```python
from build123d import *

# Parameters (mm, degrees)
F0_W     = 60
F0_H     = 15
F0_H_2   = 45
F1_DEPTH = 10
F2_DEPTH = 25
F3_DEPTH = 15
F0_W_2   = 15
F4_DEPTH = 15
F5_W     = 15
F5_H     = 15
F6_DEPTH = 20
F8_DEPTH = 40


with BuildPart() as f1:
    # F0 (on Top) → F1 (new body)
    with BuildSketch(Plane.XY):
        with Locations((0, -52.5)):
            Rectangle(F0_W, F0_H)
        with Locations((0, -22.5)):
            Rectangle(F0_W, F0_H_2)
    extrude(amount=-F1_DEPTH)

    # F0 (on Top) → F2 (join)
    with BuildSketch(Plane.XY):
        with Locations((0, -52.5)):
            Rectangle(F0_W, F0_H)
    extrude(amount=F2_DEPTH)

    # F0 (on Top) → F3 (join)
    with BuildSketch(Plane.XY):
        with Locations((0, -22.5)):
            Rectangle(F0_W, F0_H_2)
    extrude(amount=F3_DEPTH)

    # F0 (on Top) → F4 (join, through all)
    with BuildSketch(Plane.XY):
        with Locations((22.5, 52.5)):
            Rectangle(F0_W_2, F0_H)
        Polygon((15, 45), (15, 60), (-15, 60), (-15, 45), (-30, 45), (-30, 0), (30, 0), (30, 45), align=None)
        with Locations((-22.5, 52.5)):
            Rectangle(F0_W_2, F0_H)
    extrude(amount=F4_DEPTH)

    # F5 (on face) → F6 (join)
    with BuildSketch(Plane.XY.offset(15)):
        with Locations((-22.5, 52.5)):
            Rectangle(F5_W, F5_H)
        with Locations((22.5, 52.5)):
            Rectangle(F5_W, F5_H)
    extrude(amount=F6_DEPTH)

    # F7 (on face) → F8 (cut)
    with BuildSketch(Plane.XY.offset(15)):
        with BuildLine():
            ThreePointArc((10, 20), (-7.071068, 27.071068), (0, 10))
            ThreePointArc((0, 10), (7.071068, 12.928932), (10, 20))
        make_face()
        with BuildLine():
            Line((0, -25), (0, -35))
            ThreePointArc((0, -35), (7.071068, -32.071068), (10, -25))
            ThreePointArc((10, -25), (7.071068, -17.928932), (0, -15))
            Line((0, -15), (0, -25))
        make_face()
        with BuildLine():
            ThreePointArc((0, -15), (-10, -25), (0, -35))
            Line((0, -35), (0, -25))
            Line((0, -25), (0, -15))
        make_face()
    extrude(amount=-F8_DEPTH, mode=Mode.SUBTRACT)


solid = f1.part
```
For this review, take the finished solid that the model builds, in its own axes (mm). A direction names the side the tool comes from. Round coordinates to 2 decimals unless told otherwise and drop trailing zeros. Write each loop counter-clockwise with the first axis right and the second up, starting at its lowest first coordinate (ties: lowest second). Pieces come first, ordered by that corner, then holes.
1) Take a section at A-A on z = 19.5. Give the boundary of the cut face in (x, y).
Answer below:
outline: (-30, -60) - (30, -60) - (30, -45) - (-30, -45) - close; (-30, 45) - (-15, 45) - (-15, 60) - (-30, 60) - close; (15, 45) - (30, 45) - (30, 60) - (15, 60) - close
2) Machinability: for faces 5 (the face through (-23, 45, 25)), 6 (the face through (15, 52, 25)), 7 (the face through (0, -52, 25)), 8 (the face through (-0.4, 30.4, 0)), which of the approach directions +Z, -Z, +X, -X, +Y, -Y give a long, thin tool a straight path to every point of the face, cutting with its end or side? Answer none if there is none.
Answer below:
face 5: +Z, +X, -X
face 6: +Z, +Y
face 7: +Z, +X, -X, -Y
face 8: -Z, +X, -X, +Y
3) Insertion check: pin 1 Ø2 at (x, y) = (-16, -4.5) entering from +Z; pin 2 Ø16.5 at (x, y) = (-2, -52) entering from +Z; pin 3 Ø5 at (x, z) = (0.5, -3) entering from +Y. Each pin has a flat end and moves straight along its axis. Give the tip position at first contact, or say it passes through.
Answer below:
pin 1: stops at z = 15
pin 2: stops at z = 25
pin 3: stops at y = 0
4) Take a section at C-C on y = 24. Give the boundary of the cut face in (x, z), then the cut area to 3 significant figures.
Answer below:
outline: (-30, 0) - (-9.17, 0) - (-9.17, 15) - (-30, 15) - close; (9.17, 0) - (30, 0) - (30, 15) - (9.17, 15) - close
area: 625 mm2
5) Take a section at B-B on x = -5. Give the boundary of the cut face in (y, z), then the cut area to 3 significant figures.
Answer below:
outline: (-60, -10) - (-33.66, -10) - (-33.66, 15) - (-45, 15) - (-45, 25) - (-60, 25) - close; (-16.34, -10) - (0, -10) - (0, 0) - (11.34, 0) - (11.34, 15) - (-16.34, 15) - close; (28.66, 0) - (60, 0) - (60, 15) - (28.66, 15) - close
area: 1,860 mm2
6) Mouldability with a two-part tool opening along Y and no side actions: class faces 1 (the face through (22, 45, 25)), 2 (the face through (0, -45, 20)), 3 (the face through (0, -36, -10)), 4 (the face through (0, 60, 13)) as +Y half, -Y half, draft (parallel to the pull), parting line (faces both ways), or undercut.
Answer below:
face 1: undercut
face 2: undercut
face 3: draft
face 4: +Y half
7) For line 1 along X through (y, z) = (20, 3.75); line 2 along Z through (x, y) = (-6.5, -5); line 3 along Y through (x, z) = (21, 21), list the stretches that pass through material, from the lowest coordinate up.
Answer below:
line 1: x = -30 to -10, 10 to 30
line 2: z = -10 to 15
line 3: y = -60 to -45, 45 to 60
8) Take a section at D-D on x = 18. Give the boundary of the cut face in (y, z), then the cut area to 3 significant figures.
Answer below:
outline: (-60, -10) - (0, -10) - (0, 0) - (60, 0) - (60, 35) - (45, 35) - (45, 15) - (-45, 15) - (-45, 25) - (-60, 25) - close
area: 2,850 mm2
